```python
from build123d import *

# Parameters (mm, degrees)
EXTRUDE_1_DEPTH     = 20
SKETCH_2_W          = 10
SKETCH_2_H          = 19.900109324
EXTRUDE_2_DEPTH     = 30
SKETCH_3_R          = 2.5
CUT_EXTRUDE_1_DEPTH = 15
SKETCH_6_R          = 5
CUT_EXTRUDE_3_DEPTH = 9


with BuildPart() as part:
    # 草圖1 → 填料-伸長1 (new body)
    with BuildSketch(Plane(origin=(0, 0, 0), x_dir=(1, 0, 0), z_dir=(0, 1, 0))):
        with BuildLine():
            Line((18.090545138, 11.779886892), (17.195277264, 13.012117407))
            ThreePointArc((17.195277264, 13.012117407), (14.912835639, 8.338920118), (15.985777721, 3.25))
            Line((15.985777721, 3.25), (-30, 3.25))
            Line((-30, 3.25), (-30, -3.25))
            Line((-30, -3.25), (30, -3.25))
            Line((30, -3.25), (30, 3.25))
            Line((30, 3.25), (29.718485306, 3.25))
            ThreePointArc((29.718485306, 3.25), (30.775982744, 8.456436022), (28.338903699, 13.177232841))
            Line((28.338903699, 13.177232841), (27.448325592, 11.951457236))
            ThreePointArc((27.448325592, 11.951457236), (22.97128582, 0.856355384), (18.090545138, 11.779886892))
        make_face()
    extrude(amount=EXTRUDE_1_DEPTH)

    # 草圖2 → 填料-伸長2 (add)
    with BuildSketch(Plane(origin=(0, 0, -3.25), x_dir=(-1, 0, 0), z_dir=(0, 0, -1))):
        with Locations((25, 10.049945338)):
            Rectangle(SKETCH_2_W, SKETCH_2_H)
    extrude(amount=EXTRUDE_2_DEPTH)

    # 草圖3 → 除料-伸長1 (cut)
    with BuildSketch(Plane(origin=(-20, 0, 0), x_dir=(0, 0, -1), z_dir=(1, 0, 0))):
        with Locations((23.481727135, 11.991404281)):
            Circle(SKETCH_3_R)
        with Locations(Location((10.481727135, 11.991404281, 0), (0, 0, 180))):
            Circle(SKETCH_3_R)
    extrude(amount=-CUT_EXTRUDE_1_DEPTH, mode=Mode.SUBTRACT)

    # 草圖6 → 除料-伸長3 (cut)
    with BuildSketch(Plane(origin=(-20, 0, 0), x_dir=(0, 0, -1), z_dir=(1, 0, 0))):
        with Locations((23.481727135, 11.991404281)):
            Circle(SKETCH_6_R)
        with Locations(Location((10.481727135, 11.991404281, 0), (0, 0, 180))):
            Circle(SKETCH_6_R)
    extrude(amount=-CUT_EXTRUDE_3_DEPTH, mode=Mode.SUBTRACT)


solid = part.part
```
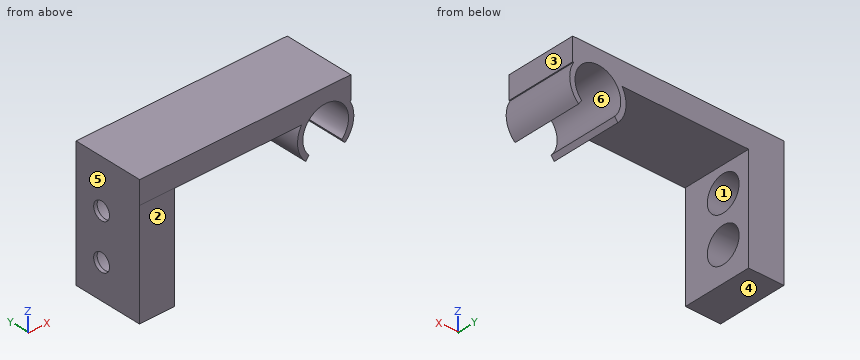
CAD build for the part. Positions are in the model's coordinates, mm. Face numbers are marked on the shaded views. A direction names the side the tool comes from. Coordinates: 2 decimals unless noted, no trailing zeros. Order: outer loops, then holes, each group sorted by start corner. A loop starts at its lowest first (then second) coordinate and runs counter-clockwise, first axis right, second up. Notation, with made-up numbers: (37.25, -5) - (88.25, -5) arc R19 ccw to (88.25, 4) - close; hole circle Ø6 at (57, -39). An arc over 180 degrees is marked (long way). Use a Markdown table: item, result. Add a question column.
(1) Which spindle directions (+Z, -Z, +X, -X, +Y, -Y) get a long thin tool onto all of the face, cutting with end or side? Do the marked faces 1, 2 and 3. Say none if no direction does.
(2) Drill centre lines: line 1 along Z through (x, y) = (-23.5, 8); line 2 along Z through (x, y) = (-22, 9); line 3 along X through (y, z) = (6.25, -29). Where is each one in solid material? Low to high. Write a range as [from, to].
(3) Flat gauge pins, fed straight in: pin 1 (3 mm diameter, centred on x = -26, z = -13.5, fed in from -Y); pin 2 (4.5 mm diameter, centred on y = 11.99, z = -23.48, fed in from -X); pin 3 (3 mm diameter, centred on y = 11, z = -25, fed in from +X); pin 4 (11.5 mm diameter, centred on y = 11.99, z = -23.48, fed in from +X). Where does each tip first touch, or does it go through?
(4) Saw through at B-B (x = -25). Give the cut face in (y, z), then the cut area to 3 significant figures.
(5) Saw through at C-C (z = -24). Give the cut face in (x, y).
(6) Pull direction Z, two halves, no side cores. Call the marked faces 4, 5 and 6: +Z half, -Z half, draft (parallel to the pull), parting line (faces both ways), or undercut.
(7) Saw through at A-A (y = 17.75). Give the cut face in (x, z).
(8) Saw through at D-D (y = 11). Give the cut face in (x, z), then the cut area to 3 significant figures.
Solved:
| question | item | result |
|---|---|---|
| 1 | face 1 | none |
| 1 | face 2 | -Z, -X, -Y |
| 1 | face 3 | +Z, +X, +Y, -Y |
| 2 | line 1 | z = [-33.25, -26.49], [-20.47, -13.49], [-7.47, 3.25] |
| 2 | line 2 | z = [-33.25, -27.49], [-19.48, -14.49], [-6.48, 3.25] |
| 2 | line 3 | x = [-30, -20] |
| 3 | pin 1 | stops at y = 0.1 |
| 3 | pin 2 | passes through |
| 3 | pin 3 | stops at x = -29 |
| 3 | pin 4 | stops at x = -20 |
| 4 | outline | (0, -3.25) - (0.1, -3.25) - (0.1, -33.25) - (20, -33.25) - (20, 3.25) - (0, 3.25) - close; hole circle Ø10 at (11.99, -23.48); hole circle Ø10 at (11.99, -10.48) |
| 4 | area | 570 mm² |
| 5 | outline | (-30, 0.1) - (-20, 0.1) - (-20, 7.02) - (-29, 7.02) - (-29, 9.55) - (-30, 9.55) - close; (-30, 14.44) - (-29, 14.44) - (-29, 16.96) - (-20, 16.96) - (-20, 20) - (-30, 20) - close |
| 6 | face 4 | -Z half |
| 6 | face 5 | draft |
| 6 | face 6 | undercut |
| 7 | outline | (-30, -33.25) - (-20, -33.25) - (-20, -3.25) - (15.99, -3.25) arc R8 ccw to (17.2, -13.01) - (18.09, -11.78) arc R6.5 cw (long way) to (27.45, -11.95) - (28.34, -13.18) arc R8 ccw to (29.72, -3.25) - (30, -3.25) - (30, 3.25) - (-30, 3.25) - close |
| 8 | outline | (-30, -33.25) - (-20, -33.25) - (-20, -28.38) - (-29, -28.38) - (-29, -25.78) - (-30, -25.78) - close; (-30, -21.19) - (-29, -21.19) - (-29, -18.58) - (-20, -18.58) - (-20, -15.38) - (-29, -15.38) - (-29, -12.78) - (-30, -12.78) - close; (-30, -8.19) - (-29, -8.19) - (-29, -5.58) - (-20, -5.58) - (-20, -3.25) - (15.99, -3.25) arc R8 ccw to (17.2, -13.01) - (18.09, -11.78) arc R6.5 cw (long way) to (27.45, -11.95) - (28.34, -13.18) arc R8 ccw to (29.72, -3.25) - (30, -3.25) - (30, 3.25) - (-30, 3.25) - close |
| 8 | area | 518 mm² |
